from build123d import *

# Parameters (mm, degrees)
F1_DEPTH = 923.925
F2_W     = 152.4
F2_H     = 215.9
F2_R     = 7.14375
F3_DEPTH = 19.05
F4_W     = 63.5
F4_H     = 381
F4_R     = 8.73125
F5_DEPTH = 66.548
F6_W     = 177.8
F6_H     = 114.3
F6_R     = 12.7
F6_W_2   = 254
F7_DEPTH = 66.548


with BuildPart() as f1:
    # F0 (on Right) → F1 (new body, symmetric)
    with BuildSketch(Plane.YZ):
        with BuildLine():
            Line((415.925, 171.45), (-415.925, 171.45))
            ThreePointArc((-415.925, 171.45), (-438.37564, 162.15064), (-447.675, 139.7))
            Line((-447.675, 139.7), (-447.675, -139.7))
            ThreePointArc((-447.675, -139.7), (-453.254616, -153.170384), (-466.725, -158.75))
            Line((-466.725, -158.75), (-574.675, -158.75))
            Line((-574.675, -158.75), (-574.675, -171.45))
            Line((-574.675, -171.45), (-466.725, -171.45))
            ThreePointArc((-466.725, -171.45), (-444.27436, -162.15064), (-434.975, -139.7))
            Line((-434.975, -139.7), (-434.975, 139.7))
            ThreePointArc((-434.975, 139.7), (-429.395384, 153.170384), (-415.925, 158.75))
            Line((-415.925, 158.75), (415.925, 158.75))
            ThreePointArc((415.925, 158.75), (429.395384, 153.170384), (434.975, 139.7))
            Line((434.975, 139.7), (434.975, -139.7))
            ThreePointArc((434.975, -139.7), (444.27436, -162.15064), (466.725, -171.45))
            Line((466.725, -171.45), (574.675, -171.45))
            Line((574.675, -171.45), (574.675, -158.75))
            Line((574.675, -158.75), (466.725, -158.75))
            ThreePointArc((466.725, -158.75), (453.254616, -153.170384), (447.675, -139.7))
            Line((447.675, -139.7), (447.675, 139.7))
            ThreePointArc((447.675, 139.7), (438.37564, 162.15064), (415.925, 171.45))
        make_face()
    extrude(amount=F1_DEPTH, both=True)

    # F2 (on face) → F3 (join)
    with BuildSketch(Plane.XY.offset(171.45)):
        with Locations((830.961, 174.625)):
            Rectangle(F2_W, F2_H)
        with Locations((783.209, 95.377)):
            Circle(F2_R, mode=Mode.SUBTRACT)
        with Locations((878.713, 95.377)):
            Circle(F2_R, mode=Mode.SUBTRACT)
        with Locations((783.209, 253.873)):
            Circle(F2_R, mode=Mode.SUBTRACT)
        with Locations((878.713, 253.873)):
            Circle(F2_R, mode=Mode.SUBTRACT)
    extrude(amount=F3_DEPTH)

    # F4 (on face) → F5 (join)
    with BuildSketch(Plane.XY.offset(171.45)):
        with Locations((491.871, 174.625)):
            Rectangle(F4_W, F4_H)
        with Locations((492.125, 73.025)):
            Circle(F4_R, mode=Mode.SUBTRACT)
        with Locations((492.125, 276.225)):
            Circle(F4_R, mode=Mode.SUBTRACT)
        with Locations((650.875, 174.625)):
            Rectangle(F4_W, F4_H)
        with Locations((650.621, 73.025)):
            Circle(F4_R, mode=Mode.SUBTRACT)
        with Locations((650.621, 276.225)):
            Circle(F4_R, mode=Mode.SUBTRACT)
    extrude(amount=F5_DEPTH)

    # F6 (on face) → F7 (join)
    with BuildSketch(Plane.XY.offset(171.45)):
        with Locations((-114.427, 3.175)):
            Rectangle(F6_W, F6_H)
        with Locations((-120.777, -3.175)):
            Circle(F6_R, mode=Mode.SUBTRACT)
        with Locations((291.973, 3.175)):
            Rectangle(F6_W_2, F6_H)
        with Locations((336.423, -3.175)):
            Circle(F6_R, mode=Mode.SUBTRACT)
        with Locations((-114.427, 346.075)):
            Rectangle(F6_W, F6_H)
        with Locations((-120.777, 352.425)):
            Circle(F6_R, mode=Mode.SUBTRACT)
        with Locations((291.973, 346.075)):
            Rectangle(F6_W_2, F6_H)
        with Locations((336.423, 352.425)):
            Circle(F6_R, mode=Mode.SUBTRACT)
    extrude(amount=F7_DEPTH)


solid = f1.part
The model under review builds one solid part; all positions refer to its coordinate system, in mm. A direction names the side the tool comes from. Round coordinates to 2 decimals unless told otherwise and drop trailing zeros. Write each loop counter-clockwise with the first axis right and the second up, starting at its lowest first coordinate (ties: lowest second). Pieces come first, ordered by that corner, then holes. Notation, with made-up numbers: M -11.5,56.5 L 13.5,56.5 A33 cw 13.5,86.5 Z; hole C -40,80.25 d11. An arc over 180 degrees is marked long. Answer as CSV lines item,"result". Start each with the question number.
Q1. Wall thickness on line 1 along Y through (x, z) = (-618.5, -100) (3 decimals); line 2 along Y through (x, z) = (203, 199) (3 decimals); line 3 along Z through (x, y) = (-838, 219): over which ranges is each line inside the solid? List them lowest first.
Q2. Consider section B-B, the plane y = 148. Give the boundary of the cut face in (x, z) (3 decimals).
Q3. Consider section A-A, the plane z = 83.5. Give the boundary of the cut face in (x, y) (3 decimals).
Q4. The part is to be moulded in two halves that separate along Y. For faces 1 (the face through (13, 434.975, 2)), 2 (the face through (650, -15.875, 204)), 3 (the face through (13, 520, -171.45)), 4 (the face through (290, 288.925, 204)), say which applies: +Y half, -Y half, draft (parallel to the pull), parting line (faces both ways), or undercut.
Q5. Consider section C-C, the plane x = 552.5. Give the boundary of the cut face in (y, z) (3 decimals), then the cut area to 3 significant figures.
Q6. Clearance check with flat-ended pins moving along their axes: P1, Ø19, axis at x = 649.5, y = 71, coming from the +Z side; P2, Ø18.5, axis at x = 878.713, y = 253.873, coming from the +Z side; P3, Ø20, axis at y = 2.5, z = 215.5, coming from the -X side; P4, Ø5, axis at x = 66.5, y = 285, coming from the -Z side. State where each tip first meets the part, or that it passes through.
Q7. Consider section D-D, the plane y = -223. Give the boundary of the cut face in (x, z) (3 decimals), then the cut area to 3 significant figures.
Q8. Tool access review of faces 5 (the face through (-116, 403.225, 204)), 6 (the face through (164.973, 345, 204)), 7 (the face through (13, -520, -158.75)): name each direction out of +Z, -Z, +X, -X, +Y, -Y from which nothing blocks a thin tool from reaching the whole face with its end or side.
Result set:
1,line 1,"y = -447.675 to -434.975, 434.975 to 447.675"
1,line 2,"y = -53.975 to 60.325, 288.925 to 403.225"
1,line 3,"z = 158.75 to 171.45"
2,outline,"M -923.925,158.75 L 923.925,158.75 L 923.925,171.45 L 907.161,171.45 L 907.161,190.5 L 754.761,190.5 L 754.761,171.45 L 682.625,171.45 L 682.625,237.998 L 619.125,237.998 L 619.125,171.45 L 523.621,171.45 L 523.621,237.998 L 460.121,237.998 L 460.121,171.45 L -923.925,171.45 Z"
3,outline,"M -923.925,-447.675 L 923.925,-447.675 L 923.925,-434.975 L -923.925,-434.975 Z; M -923.925,434.975 L 923.925,434.975 L 923.925,447.675 L -923.925,447.675 Z"
4,face 1,"undercut"
4,face 2,"-Y half"
4,face 3,"draft"
4,face 4,"undercut"
5,outline,"M -574.675,-171.45 L -466.725,-171.45 A31.75 ccw -434.975,-139.7 L -434.975,139.7 A19.05 cw -415.925,158.75 L 415.925,158.75 A19.05 cw 434.975,139.7 L 434.975,-139.7 A31.75 ccw 466.725,-171.45 L 574.675,-171.45 L 574.675,-158.75 L 466.725,-158.75 A19.05 cw 447.675,-139.7 L 447.675,139.7 A31.75 ccw 415.925,171.45 L -415.925,171.45 A31.75 ccw -447.675,139.7 L -447.675,-139.7 A19.05 cw -466.725,-158.75 L -574.675,-158.75 Z"
5,area,"22,400 mm²"
6,P1,"stops at z = 238"
6,P2,"stops at z = 190.5"
6,P3,"stops at x = -203.33"
6,P4,"stops at z = 158.75"
7,outline,"M -923.925,158.75 L 923.925,158.75 L 923.925,171.45 L -923.925,171.45 Z"
7,area,"23,500 mm²"
8,face 5,"+Z, +X, -X, +Y"
8,face 6,"+Z, +Y, -Y"
8,face 7,"+Z, +X, -X, -Y"
